```python
from build123d import *

# Parameters (mm, degrees)
SKETCH2_R           = 5.1
SKETCH2_R_2         = 2.7
BOSS_EXTRUDE1_DEPTH = 2
SKETCH3_R           = 4
SKETCH3_R_2         = 2.7
BOSS_EXTRUDE2_DEPTH = 19
SKETCH4_R           = 5.1
SKETCH4_R_2         = 2.7
BOSS_EXTRUDE3_DEPTH = 2
CHAMFER1_SIZE       = 1.2
CHAMFER2_SIZE       = 0.5


with BuildPart() as part:
    # Sketch2 → Boss-Extrude1 (new body)
    with BuildSketch(Plane.XY):
        Circle(SKETCH2_R)
        Circle(SKETCH2_R_2, mode=Mode.SUBTRACT)
    extrude(amount=BOSS_EXTRUDE1_DEPTH)

    # Sketch3 → Boss-Extrude2 (add)
    with BuildSketch(Plane.XY.offset(2)):
        Circle(SKETCH3_R)
        Circle(SKETCH3_R_2, mode=Mode.SUBTRACT)
    extrude(amount=BOSS_EXTRUDE2_DEPTH)

    # Sketch4 → Boss-Extrude3 (add)
    with BuildSketch(Plane.XY.offset(21)):
        Circle(SKETCH4_R)
        Circle(SKETCH4_R_2, mode=Mode.SUBTRACT)
    extrude(amount=BOSS_EXTRUDE3_DEPTH)

    # Chamfer1
    # the kernel refuses this chamfer: 1.2 mm, written as the material it adds along each edge
    with BuildSketch(Plane(origin=(0, 0, 21), x_dir=(1, 0, 0), z_dir=(0, -1, 0))) as chamfer1_piece_1_section:
        Polygon((4, -CHAMFER1_SIZE), (4 + CHAMFER1_SIZE, 0), (4, 0), align=None)
    chamfer1_piece_1 = revolve(axis=Axis((0, 0, 21), (0, 0, 1)), mode=Mode.PRIVATE)
    chamfer1_piece_1 = chamfer1_piece_1 & Plane(origin=(0, 0, 20.352695211), x_dir=(1, 0, 0), z_dir=(0, 0, -1)) * Cylinder(5.1, 21, mode=Mode.PRIVATE)
    add(chamfer1_piece_1)
    with BuildSketch(Plane(origin=(0, 0, 2), x_dir=(1, 0, 0), z_dir=(0, -1, 0))) as chamfer1_piece_2_section:
        Polygon((4 + CHAMFER1_SIZE, 0), (4, CHAMFER1_SIZE), (4, 0), align=None)
    chamfer1_piece_2 = revolve(axis=Axis((0, 0, 2), (0, 0, 1)), mode=Mode.PRIVATE)
    chamfer1_piece_2 = chamfer1_piece_2 & Plane(origin=(0, 0, 2.647304789), x_dir=(1, 0, 0), z_dir=(0, 0, -1)) * Cylinder(5.1, 21, mode=Mode.PRIVATE)
    add(chamfer1_piece_2)

    # Chamfer2
    chamfer2_edges = [part.edges().sort_by_distance(p)[0] for p in [
        (-2.7, 0, 23),
        (-2.7, 0, 0),
    ]]
    chamfer(chamfer2_edges, length=CHAMFER2_SIZE)


solid = part.part
```
Source: CAD feature listing. Evaluate the final solid. Frame: model axes, mm. A direction names the side the tool comes from. Give positions to 0.01 mm unless a question says otherwise; leave off trailing zeros. Loops run counter-clockwise (first coordinate to the right, second up) from the corner with the lowest first, then second, coordinate; pieces in that order, holes last. Notation, with made-up numbers: (63.5, 38) -> (108.5, 38) arc R26 cw to (108.5, 61) -> close; hole circle Ø11 at (50.25, 44). An arc over 180 degrees is marked (long way). Use a Markdown table: item, result. Add a question column.
(1) Access query for faces 4 (the face through (3.3, -1.1, 0)), 5 (the face through (-0.867, -3.905, 11.384)). Directions: +Z, -Z, +X, -X, +Y, -Y. A direction counts if a zero-diameter tool reaches every point of the face in a straight line with its end or side. Return the directions, or none.
(2) Ray query, line 1 (Y direction, x = 0, z = 6.25); line 2 (X direction, y = -1.25, z = 21.25); line 3 (Z direction, x = 4, y = -1). Return the intervals inside material, ascending.
(3) Section query C-C (z = 13.5). Output: boundary loops of the cut face in (x, y).
(4) Section query A-A (x = 0). Output: boundary loops of the cut face in (y, z), then the cut area to 3 significant figures.
(5) Pull-direction query (Y, two-part tool) for faces 1 (the face through (3.3, -1.1, 23)), 2 (the face through (-0.585, -2.636, 11.346)), 3 (the face through (2.4, 4.5, 21.9)); classes: +Y half, -Y half, draft (parallel to the pull), parting line (faces both ways), or undercut.
(6) First-contact query: pin 1 Ø6 at (y, z) = (1, 17) entering from +X; pin 2 Ø1 at (x, y) = (-0.5, 1) entering from +Z; pin 3 Ø3 at (y, z) = (3, 10) entering from +X; pin 4 Ø2 at (x, z) = (-3.5, 19.5) entering from +Y. Flat tips, straight axial feed; report the tip coordinate or a pass-through.
Checked values:
| question | item | result |
|---|---|---|
| 1 | face 4 | -Z, +X, -X, +Y, -Y |
| 1 | face 5 | none |
| 2 | line 1 | -4 to -2.7, 2.7 to 4 |
| 2 | line 2 | -4.94 to -2.39, 2.39 to 4.94 |
| 2 | line 3 | 0 to 3.08, 19.92 to 23 |
| 3 | outline | circle Ø8 at (0, 0); hole circle Ø5.4 at (0, 0) |
| 4 | outline | (-5.1, 0) -> (-3.2, 0) -> (-2.7, 0.5) -> (-2.7, 22.5) -> (-3.2, 23) -> (-5.1, 23) -> (-5.1, 20.9) -> (-4, 19.8) -> (-4, 3.2) -> (-5.1, 2.1) -> close; (2.7, 0.5) -> (3.2, 0) -> (5.1, 0) -> (5.1, 2.1) -> (4, 3.2) -> (4, 19.8) -> (5.1, 20.9) -> (5.1, 23) -> (3.2, 23) -> (2.7, 22.5) -> close |
| 4 | area | 71.0 mm^2 |
| 5 | face 1 | draft |
| 5 | face 2 | undercut |
| 5 | face 3 | parting line |
| 6 | pin 1 | x = 4.13 |
| 6 | pin 2 | through |
| 6 | pin 3 | x = 3.71 |
| 6 | pin 4 | y = 3.44 |
